Check sheet for the drawn part. Datum: minimum x, y, z corner. Units: mm. Round coordinates to 2 decimals unless told otherwise and drop trailing zeros. Write each loop counter-clockwise with the first axis right and the second up, starting at its lowest first coordinate (ties: lowest second). Pieces come first, ordered by that corner, then holes. Notation, with made-up numbers: (8.25, 21.25) - (44.25, 21.25) arc R19 ccw to (44.25, 54.25) - close; hole circle Ø9 at (20, 83.5). An arc over 180 degrees is marked (long way). Answer as a JSON object with one key per item and string values. Group by question number.
1) Go/stop test with flat-tipped pins: pin 1 Ø1.4 at (x, y) = (1.5, 18) entering from -Z (3 decimals); pin 2 Ø2.5 at (x, z) = (1.5, 116) entering from +Y; pin 3 Ø1.4 at (x, y) = (3.5, 1.5) entering from -Z (3 decimals). Record where each tip stops, or that it passes through.
2) Section check B-B (x = 2.75). Enter the section's corners in (y, z) (3 decimals).
3) Section check A-A (y = 18). Enter the section's corners in (x, z) (3 decimals), then the cut area to 3 significant figures.
4) Section check C-C (z = 104.5). Enter the section's corners in (x, y), then the cut area to 3 significant figures.
5) Thickness scan on line 1 (Z direction, x = 4.35, y = 15.5) (3 decimals); line 2 (Z direction, x = 3.55, y = 4) (3 decimals); line 3 (Y direction, x = 0.4, z = 20.5). Record the ranges inside material, lowest first.
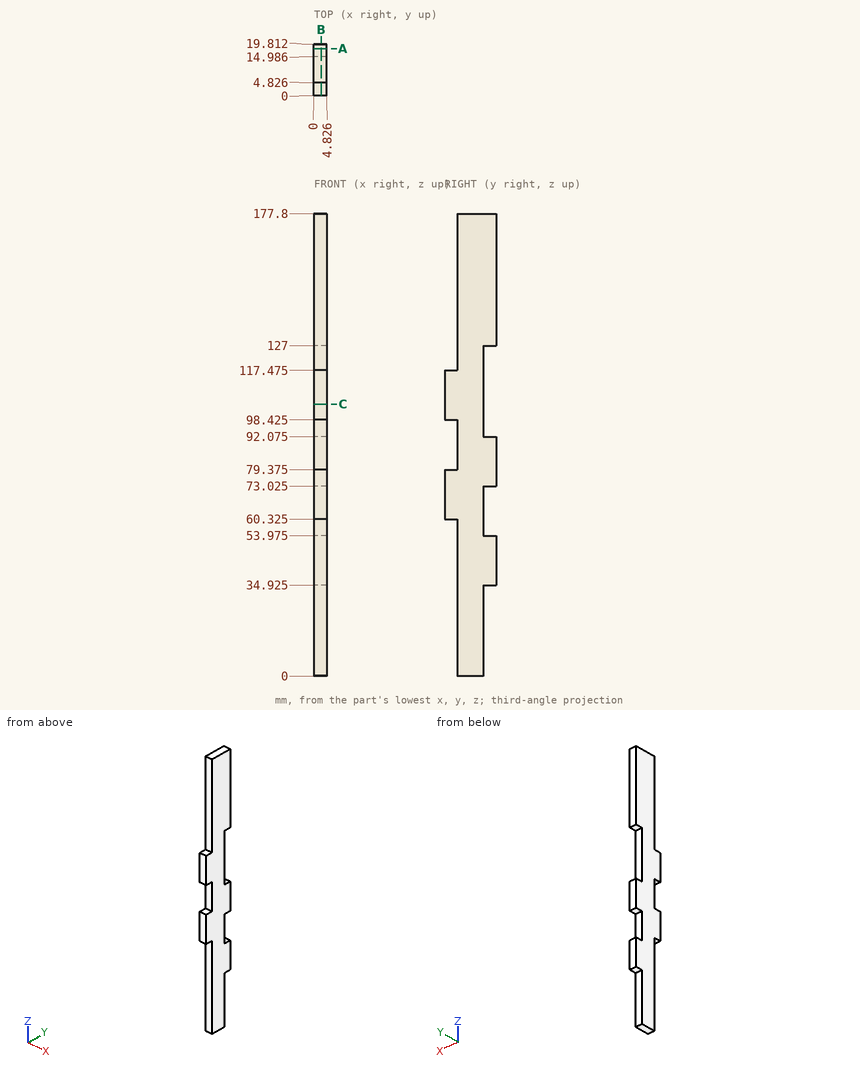
Returned:
{
 "1": {"pin 1": "z = 34.925", "pin 2": "y = 14.99", "pin 3": "z = 60.325"},
 "2": {"outline": "(0, 60.325) - (4.826, 60.325) - (4.826, 0) - (14.986, 0) - (14.986, 34.925) - (19.812, 34.925) - (19.812, 53.975) - (14.986, 53.975) - (14.986, 73.025) - (19.812, 73.025) - (19.812, 92.075) - (14.986, 92.075) - (14.986, 127) - (19.812, 127) - (19.812, 177.8) - (4.826, 177.8) - (4.826, 117.475) - (0, 117.475) - (0, 98.425) - (4.826, 98.425) - (4.826, 79.375) - (0, 79.375) - close"},
 "3": {"outline": "(0, 34.925) - (4.826, 34.925) - (4.826, 53.975) - (0, 53.975) - close; (0, 73.025) - (4.826, 73.025) - (4.826, 92.075) - (0, 92.075) - close; (0, 127) - (4.826, 127) - (4.826, 177.8) - (0, 177.8) - close", "area": "429 mm2"},
 "4": {"outline": "(0, 0) - (4.83, 0) - (4.83, 14.99) - (0, 14.99) - close", "area": "72.3 mm2"},
 "5": {"line 1": "34.925 to 53.975, 73.025 to 92.075, 127 to 177.8", "line 2": "60.325 to 79.375, 98.425 to 117.475", "line 3": "4.83 to 14.99"}
}
